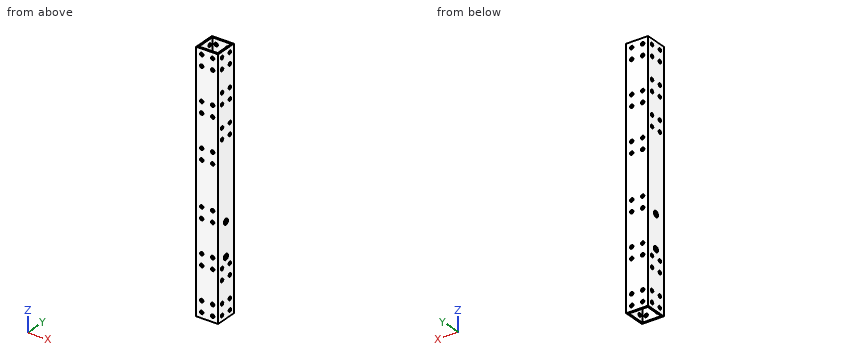
from build123d import *

# Parameters (mm, degrees)
SKETCH_1_W          = 20
SKETCH_1_H          = 20
SKETCH_1_W_2        = 17
SKETCH_1_H_2        = 17
EXTRUDE_1_DEPTH     = 230
SKETCH_2_R          = 2.65
SKETCH_2_R_2        = 1.6
CUT_EXTRUDE_1_DEPTH = 232.732604525
SKETCH_3_R          = 1.575
CUT_EXTRUDE_2_DEPTH = 232.732604525


with BuildPart() as part:
    # 草图1 → 拉伸-薄壁1 (new body)
    with BuildSketch(Plane.XY):
        with Locations((10, -10)):
            Rectangle(SKETCH_1_W, SKETCH_1_H)
        with Locations((10, -10)):
            Rectangle(SKETCH_1_W_2, SKETCH_1_H_2, mode=Mode.SUBTRACT)
    extrude(amount=EXTRUDE_1_DEPTH)

    # 草图2 → 切除-拉伸1 (cut, through all)
    with BuildSketch(Plane(origin=(20, 0, 0), x_dir=(0, 0, -1), z_dir=(1, 0, 0))):
        with Locations((-82.7, -10)):
            Circle(SKETCH_2_R)
        with Locations((-52.7, -10)):
            Circle(SKETCH_2_R)
        with Locations((-225, -5)):
            Circle(SKETCH_2_R_2)
        with Locations(Location((-225, -15, 0), (0, 0, 180))):
            Circle(SKETCH_2_R_2)
        with Locations((-215, -15)):
            Circle(SKETCH_2_R_2)
        with Locations(Location((-215, -5, 0), (0, 0, 180))):
            Circle(SKETCH_2_R_2)
        with Locations((-195, -5)):
            Circle(SKETCH_2_R_2)
        with Locations(Location((-185, -5, 0), (0, 0, 180))):
            Circle(SKETCH_2_R_2)
        with Locations((-185, -15)):
            Circle(SKETCH_2_R_2)
        with Locations(Location((-195, -15, 0), (0, 0, 180))):
            Circle(SKETCH_2_R_2)
        with Locations((-165, -5)):
            Circle(SKETCH_2_R_2)
        with Locations(Location((-155, -5, 0), (0, 0, 180))):
            Circle(SKETCH_2_R_2)
        with Locations((-155, -15)):
            Circle(SKETCH_2_R_2)
        with Locations(Location((-165, -15, 0), (0, 0, 180))):
            Circle(SKETCH_2_R_2)
        with Locations((-35, -15)):
            Circle(SKETCH_2_R_2)
        with Locations(Location((-45, -15, 0), (0, 0, 180))):
            Circle(SKETCH_2_R_2)
        with Locations((-45, -5)):
            Circle(SKETCH_2_R_2)
        with Locations(Location((-35, -5, 0), (0, 0, 180))):
            Circle(SKETCH_2_R_2)
        with Locations((-15, -5)):
            Circle(SKETCH_2_R_2)
        with Locations(Location((-15, -15, 0), (0, 0, 180))):
            Circle(SKETCH_2_R_2)
        with Locations((-5, -15)):
            Circle(SKETCH_2_R_2)
        with Locations(Location((-5, -5, 0), (0, 0, 180))):
            Circle(SKETCH_2_R_2)
    extrude(amount=-CUT_EXTRUDE_1_DEPTH, mode=Mode.SUBTRACT)

    # 草图3 → 切除-拉伸2 (cut, through all)
    with BuildSketch(Plane(origin=(0, 0, 0), x_dir=(1, 0, 0), z_dir=(0, 1, 0))):
        with Locations(Location((5, -5, 0), (0, 0, 270))):
            Circle(SKETCH_3_R)
        with Locations(Location((15, -5, 0), (0, 0, 90))):
            Circle(SKETCH_3_R)
        with Locations(Location((15, -15, 0), (0, 0, 270))):
            Circle(SKETCH_3_R)
        with Locations(Location((5, -15, 0), (0, 0, 90))):
            Circle(SKETCH_3_R)
        with Locations(Location((5, -215, 0), (0, 0, 270))):
            Circle(SKETCH_3_R)
        with Locations(Location((15, -215, 0), (0, 0, 90))):
            Circle(SKETCH_3_R)
        with Locations(Location((15, -225, 0), (0, 0, 270))):
            Circle(SKETCH_3_R)
        with Locations(Location((5, -225, 0), (0, 0, 90))):
            Circle(SKETCH_3_R)
        with Locations(Location((5, -45, 0), (0, 0, 270))):
            Circle(SKETCH_3_R)
        with Locations(Location((15, -45, 0), (0, 0, 90))):
            Circle(SKETCH_3_R)
        with Locations(Location((15, -55, 0), (0, 0, 270))):
            Circle(SKETCH_3_R)
        with Locations(Location((5, -55, 0), (0, 0, 90))):
            Circle(SKETCH_3_R)
        with Locations(Location((5, -85, 0), (0, 0, 270))):
            Circle(SKETCH_3_R)
        with Locations(Location((15, -85, 0), (0, 0, 90))):
            Circle(SKETCH_3_R)
        with Locations(Location((15, -95, 0), (0, 0, 270))):
            Circle(SKETCH_3_R)
        with Locations(Location((5, -95, 0), (0, 0, 90))):
            Circle(SKETCH_3_R)
        with Locations(Location((5, -135, 0), (0, 0, 270))):
            Circle(SKETCH_3_R)
        with Locations(Location((15, -135, 0), (0, 0, 90))):
            Circle(SKETCH_3_R)
        with Locations(Location((15, -145, 0), (0, 0, 270))):
            Circle(SKETCH_3_R)
        with Locations(Location((5, -145, 0), (0, 0, 90))):
            Circle(SKETCH_3_R)
        with Locations(Location((5, -175, 0), (0, 0, 270))):
            Circle(SKETCH_3_R)
        with Locations(Location((15, -175, 0), (0, 0, 90))):
            Circle(SKETCH_3_R)
        with Locations(Location((15, -185, 0), (0, 0, 270))):
            Circle(SKETCH_3_R)
        with Locations(Location((5, -185, 0), (0, 0, 90))):
            Circle(SKETCH_3_R)
    extrude(amount=-CUT_EXTRUDE_2_DEPTH, mode=Mode.SUBTRACT)


solid = part.part
The model under review builds one solid part; all positions refer to its coordinate system, in mm. Give positions to 0.01 mm unless a question says otherwise; leave off trailing zeros. Order: outer loops, then holes, each group sorted by start corner. A loop starts at its lowest first (then second) coordinate and runs counter-clockwise, first axis right, second up. Notation, with made-up numbers: M -15.5,15.5 L -9.5,15.5 A25 cw -9.5,41.5 Z; hole C 78.25,12 d9. An arc over 180 degrees is marked long. Use one line per item in the form item = value. Start each with the question number.
Item 1: We need section A-A on x = 10. Give the boundary of the cut face in (y, z), plus the area to 3 significant figures.
Item 2: We need section B-B on z = 130. Give the boundary of the cut face in (x, y).
Item 3: To check wall thickness, follow line 1 along X through (y, z) = (-0.8, 15) (3 decimals); line 2 along Y through (x, z) = (1.05, 215); line 3 along X through (y, z) = (-7.5, 196). State the ranges of each line that lie inside material, in increasing order. Write a range as from..to.
Item 4: Insertion check: pin 1 Ø2.5 at (x, z) = (15, 185) entering from +Y. The pin has a flat end and moves straight along its axis. Give the tip position at first contact, or say it passes through.
Completed:
q1.outline = M -20,0 L -18.5,0 L -18.5,230 L -20,230 Z; M -1.5,0 L 0,0 L 0,230 L -1.5,230 Z
q1.area = 690 mm²
q2.outline = M 0,-20 L 20,-20 L 20,0 L 0,0 Z; hole M 1.5,-18.5 L 18.5,-18.5 L 18.5,-1.5 L 1.5,-1.5 Z
q3.line_1 = 0..3.425, 6.575..13.425, 16.575..20
q3.line_2 = -20..-16.6, -13.4..-6.6, -3.4..0
q3.line_3 = 0..1.5, 18.5..20
q4.pin_1 = through
